Answer from the drawing. Dimensions are ordinates in mm from the lowest x, y and z of the part. Coordinates: 2 decimals unless noted, no trailing zeros. Order: outer loops, then holes, each group sorted by start corner. A loop starts at its lowest first (then second) coordinate and runs counter-clockwise, first axis right, second up. Notation, with made-up numbers: (-22.75, 9.25) -> (8.25, 9.25) arc R19 ccw to (8.25, 15.25) -> close; hole circle Ø5 at (-16, 53). An arc over 180 degrees is marked (long way). Answer in a Markdown table with one row per item.
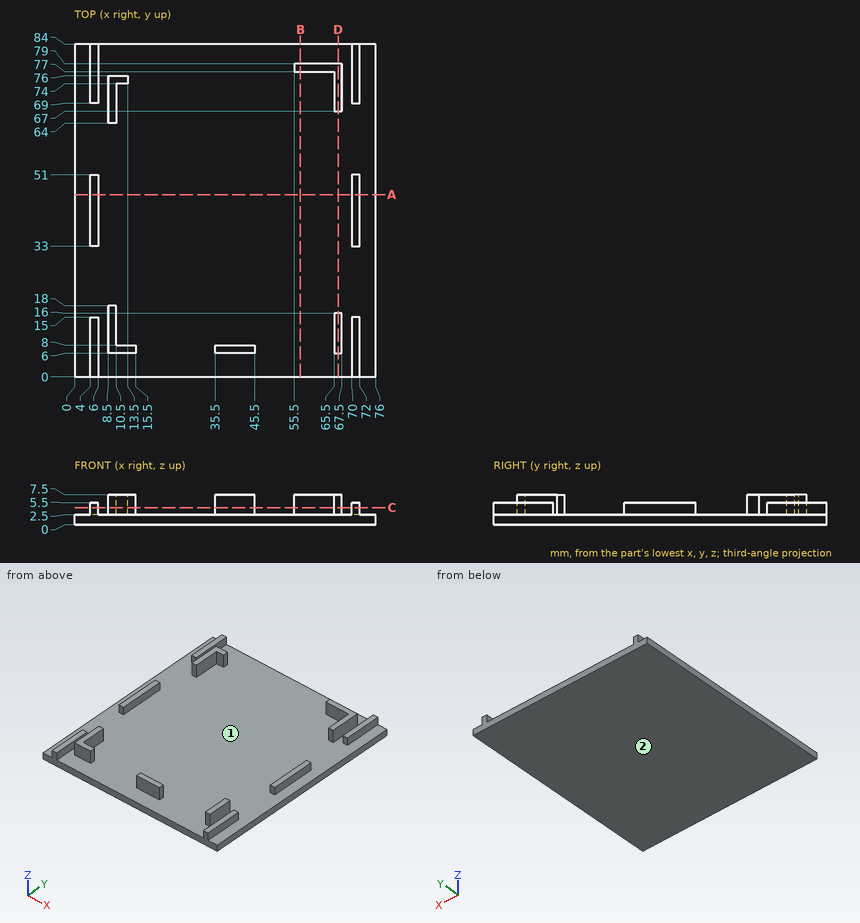
Q1. The part is cut by section C-C (z = 4.25). Give the number of separate pieces and of enclosed holes in the cut face, then the cut area to 3 significant figures.
Outcome:
| item | result |
|---|---|
| separate pieces | 11 |
| enclosed holes | 0 |
| area | 340 mm² |
Q2. Consider line 1 (X direction, y = 73, z = 4.5); line 2 (X direction, y = 39.5, z = 3.25); line 3 (Y direction, x = 5.5, z = 5). Determine where each line is inside the solid, lowest interval first.
Outcome:
| item | result |
|---|---|
| line 1 | 4 to 6, 8.5 to 10.5, 65.5 to 67.5, 70 to 72 |
| line 2 | 4 to 6, 70 to 72 |
| line 3 | 0 to 15, 33 to 51, 69 to 84 |
Q3. The part is cut by section D-D (x = 66.5). Write down the section's boundary in (y, z), then the cut area to 3 significant figures.
Outcome:
| item | result |
|---|---|
| outline | (0, 0) -> (84, 0) -> (84, 2.5) -> (79, 2.5) -> (79, 7.5) -> (67, 7.5) -> (67, 2.5) -> (16, 2.5) -> (16, 7.5) -> (6, 7.5) -> (6, 2.5) -> (0, 2.5) -> close |
| area | 320 mm² |
Q4. The part is cut by section B-B (x = 57). Write down the section's boundary in (y, z).
Outcome:
| item | result |
|---|---|
| outline | (0, 0) -> (84, 0) -> (84, 2.5) -> (79, 2.5) -> (79, 7.5) -> (77, 7.5) -> (77, 2.5) -> (0, 2.5) -> close |
Q5. Given pin 1 (3.5 mm diameter, centred on x = 12.5, z = 5.5, fed in from -Y); pin 2 (6 mm diameter, centred on x = 61.5, y = 19.5, fed in from -Z); pin 3 (1 mm diameter, centred on y = 78, z = 4.5, fed in from -X); pin 4 (2.5 mm diameter, centred on y = 7.5, z = 4, fed in from +X), each flat-ended and moving along its own axis, determine where each tip first touches the part or whether it passes through.
Outcome:
| item | result |
|---|---|
| pin 1 | y = 6 |
| pin 2 | z = 0 |
| pin 3 | x = 4 |
| pin 4 | x = 72 |
Q6. For a pull along X with two mould halves and no side action, classify the marked faces 1 and 2 as pulls with the +X half, pulls with the -X half, needs draft (parallel to the pull), parting line crosses it, or undercut.
Outcome:
| item | result |
|---|---|
| face 1 | undercut |
| face 2 | needs draft |
Q7. The part is cut by section A-A (y = 46). Write down the section's boundary in (x, z), then the cut area to 3 significant figures.
Outcome:
| item | result |
|---|---|
| outline | (0, 0) -> (76, 0) -> (76, 2.5) -> (72, 2.5) -> (72, 5.5) -> (70, 5.5) -> (70, 2.5) -> (6, 2.5) -> (6, 5.5) -> (4, 5.5) -> (4, 2.5) -> (0, 2.5) -> close |
| area | 202 mm² |
